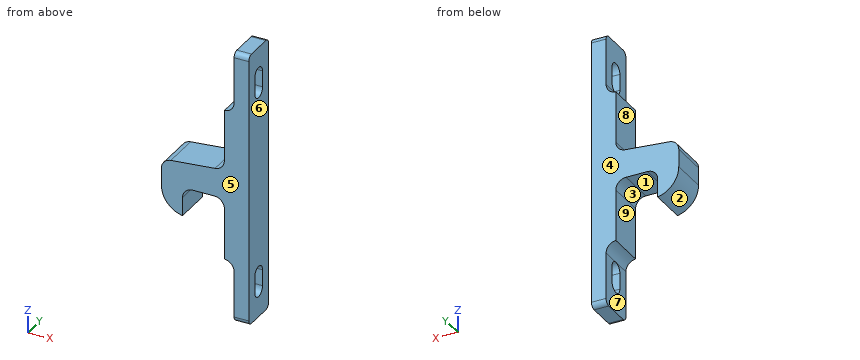
Autodesk Inventor part; units mm, degrees
ref_plane "YZ Plane" through (0, 0, 0) normal (1, 0, 0) x (0, 1, 0)
ref_plane "XZ Plane" through (0, 0, 0) normal (0, 1, 0) x (-1, 0, 0)
ref_plane "XY Plane" through (0, 0, 0) normal (0, 0, 1) x (1, 0, 0)
sketch "Boceto1" plane through (0, 0, 0) normal (0, 1, 0) x (-1, 0, 0)
  line L0 (-2.375, -26.75) -> (2.375, -26.75)
  line L1 (2.375, -26.75) -> (2.375, 26.75)
  line L2 (2.375, 26.75) -> (-2.375, 26.75)
  line L3 (-2.375, 26.75) -> (-2.375, -26.75)
  line L4 (-2.375, -26.75) -> (2.375, 26.75) construction
  line L5 (2.375, -26.75) -> (-2.375, 26.75) construction
  line L6 (2.375, 26.75) -> (0.475, 26.75)
  line L7 (0.475, 26.75) -> (0.475, 14.75)
  line L8 (0.475, 14.75) -> (2.375, 14.75)
  line L9 (2.375, 14.75) -> (2.375, 26.75)
  line L10 (2.375, -26.75) -> (0.475, -26.75)
  line L11 (0.475, -26.75) -> (0.475, -14.75)
  line L12 (0.475, -14.75) -> (2.375, -14.75)
  line L13 (2.375, -14.75) -> (2.375, -26.75)
  line L14 (2.375, -26.75) -> (2.375, -2.75)
  line L15 (2.375, -2.75) -> (10.525, -2.75)
  line L16 (10.525, -2.75) -> (10.525, -8.35)
  line L17 (10.525, -8.35) -> (14.625, -8.35)
  line L18 (14.625, -8.35) -> (14.625, 1.85)
  line L19 (14.625, 1.85) -> (2.375, 1.85)
  line L20 (14.625, 1.85) -> (2.375, 2.9217)
  point P0 (0, 0)
  point P1 (2.375, 14.75)
  point P2 (0.475, -26.75)
  point P3 (2.375, -14.75)
  dimension "d0" = 4.75
  dimension "d1" = 53.5
  dimension "d2" = 1.9
  dimension "d3" = 12
  dimension "d4" = 12
  dimension "d5" = 24
  dimension "d6" = 8.15
  dimension "d7" = 5.6
  dimension "d8" = 4.1
  dimension "d9" = 10.2
  dimension "d10" = 5
extrude "Extrusión1" add sketch "Boceto1" along normal blind 7.25 contours L3 L2 L7 L8 L1 L12 L11 L0 | L1 L19 L18 L17 L16 L15 | L1 L20 L19
fillet "Empalme1" radius 2 5 edges at (-0.475, 3.625, -14.75) (-2.375, 3.625, -2.75) (-10.525, 3.625, -2.75) (-2.375, 3.625, 2.9217) (-0.475, 3.625, 14.75)
fillet "Empalme2" radius 2 1 edges at (-14.625, 3.625, 1.85)
fillet "Empalme3" radius 5 1 edges at (-14.625, 3.625, -8.35)
fillet "Empalme4" radius 1 4 edges at (0.95, 7.25, 26.75) (0.95, 0, 26.75) (0.95, 7.25, -26.75) (0.95, 0, -26.75)
sketch "Boceto2" plane through (-0.475, 0, 16.7475) normal (-1, 0, 0) x (0, 0, 1)
  arc A0 (9.0025, 0) -> (10.0025, 1) centre (9.0025, 1) ccw
  line L0 (10.0025, 1) -> (10.0025, 6.25)
  arc A1 (10.0025, 6.25) -> (9.0025, 7.25) centre (9.0025, 6.25) ccw
  line L1 (0, 7.25) -> (9.0025, 7.25)
  line L2 (0, 0) -> (0, 7.25)
  line L3 (0, 0) -> (9.0025, 0)
  arc A2 (-43.4975, 1) -> (-42.4975, 0) centre (-42.4975, 1) ccw
  line L4 (-42.4975, 0) -> (-33.495, 0)
  line L5 (-33.495, 7.25) -> (-33.495, 0)
  line L6 (-42.4975, 7.25) -> (-33.495, 7.25)
  arc A3 (-42.4975, 7.25) -> (-43.4975, 6.25) centre (-42.4975, 6.25) ccw
  line L7 (-43.4975, 1) -> (-43.4975, 6.25)
  line L8 (4.715, 2.2) -> (2.9125, 2.2)
  line L9 (2.2, 5.05) -> (4.5775, 5.05)
  line L10 (10.0025, 3.4658) -> (6.0025, 3.4658)
  line L11 (6.0025, 3.4658) -> (6.0025, 4.2)
  line L12 (6.0025, 3.4658) -> (6.0025, 5.05)
  line L13 (4.5775, 2.2) -> (1.4275, 2.2)
  line L14 (0.0025, 3.625) -> (0.0025, 3.625)
  line L15 (1.4275, 5.05) -> (6.0025, 5.05)
  line L16 (6.0025, 3.625) -> (6.0025, 3.625)
  arc A4 (4.5775, 2.2) -> (6.0025, 3.625) centre (4.5775, 3.625) ccw
  arc A5 (6.0025, 3.625) -> (4.5775, 5.05) centre (4.5775, 3.625) ccw
  arc A6 (1.4275, 5.05) -> (0.0025, 3.625) centre (1.4275, 3.625) ccw
  arc A7 (0.0025, 3.625) -> (1.4275, 2.2) centre (1.4275, 3.625) ccw
  point P0 (-16.7475, 0)
  point P1 (6.0025, 2.2)
  point P2 (0.0025, 5.05)
  point P3 (3.715, 5.05)
  point P4 (0.0025, 3.625)
  point P5 (2.9125, 2.2)
  point P6 (4.5775, 2.2)
  point P7 (2.2, 5.05)
  dimension "d17" = 2.2
  dimension "d18" = 4
  dimension "d19" = 6
  dimension "d21" = 2.85
  dimension "d22" = 1.425
extrude "Extrusión2" cut sketch "Boceto2" against normal blind 7.25 contours L8 L13 A7 A6 L15 L9 A5 A4
ref_plane "Plano de trabajo1" through (2.375, 1, 0) normal (0, 0, -1) x (-1, 0, 0)
mirror "Simetría1" about plane through (2.375, 1, 0) normal (0, 0, -1) of "Extrusión2"
properties part number "Cierre cocina"
The model under review builds one solid part; all positions refer to its coordinate system, in mm. Face numbers are marked on the shaded views. A direction names the side the tool comes from. Give positions to 0.01 mm unless a question says otherwise; leave off trailing zeros. Loops run counter-clockwise (first coordinate to the right, second up) from the corner with the lowest first, then second, coordinate; pieces in that order, holes last. Notation, with made-up numbers: (22, -20.75) -> (74, -20.75) arc R23 cw to (74, -8.75) -> close; hole circle Ø9 at (11.5, 13.25). An arc over 180 degrees is marked (long way). Write each question's results on one line, items separated by ' | '.
1) Take a section at C-C, the plane z = 22. Give the boundary of the cut face in (x, y) (3 decimals).
Conclusion:
outline: (-0.475, 0) -> (2.375, 0) -> (2.375, 2.37) -> (-0.475, 2.37) -> close; (-0.475, 4.88) -> (2.375, 4.88) -> (2.375, 7.25) -> (-0.475, 7.25) -> close
2) Take a section at D-D, the plane x = -11. Give the boundary of the cut face in (y, z).
Conclusion:
outline: (0, -8.24) -> (7.25, -8.24) -> (7.25, 2.17) -> (0, 2.17) -> close
3) Draft analysis for pull direction X (two halves, no side actions). For the marked faces 1, 2, 3 and 4, state which applies: pulls with the +X half, pulls with the -X half, needs draft (parallel to the pull), parting line crosses it, or undercut.
Conclusion:
face 1: undercut | face 2: pulls with the -X half | face 3: undercut | face 4: needs draft
4) Insertion check: pin 1 Ø2 at (x, y) = (-4.5, 4) entering from +Z; pin 2 Ø1.2 at (x, y) = (-5.5, 5) entering from -Z; pin 3 Ø3.5 at (y, z) = (5, 20) entering from -X (3 decimals). Each pin has a flat end and moves straight along its axis. Give the tip position at first contact, or say it passes through.
Conclusion:
pin 1: stops at z = 2.96 | pin 2: stops at z = -2.75 | pin 3: stops at x = -0.475
5) Tool access review of the marked faces 5, 6, 7, 8 and 9: name each direction out of +Z, -Z, +X, -X, +Y, -Y from which nothing blocks a thin tool from reaching the whole face with its end or side.
Conclusion:
face 5: +Z, -Z, +X, -X, -Y | face 6: +Z, -Z, +X, +Y, -Y | face 7: -Z, -X, +Y, -Y | face 8: +Z, -X, +Y, -Y | face 9: -Z, +Y, -Y
6) Take a section at A-A, the plane z = -19.5. Give the boundary of the cut face in (x, y) (3 decimals), plus the area to 3 significant figures.
Conclusion:
outline: (-0.475, 0) -> (2.375, 0) -> (2.375, 2.2) -> (-0.475, 2.2) -> close; (-0.475, 5.05) -> (2.375, 5.05) -> (2.375, 7.25) -> (-0.475, 7.25) -> close | area: 12.5 mm^2
7) For line 1 along Y through (x, z) = (1.25, 18.5); line 2 along X through (y, z) = (3.5, -13) (3 decimals); line 3 along X through (y, z) = (5.25, 17.5) (3 decimals), list the stretches that pass through material, from the lowest coordinate up. Write a range as from..to.
Conclusion:
line 1: y = 0..2.2, 5.05..7.25 | line 2: x = -2.375..2.375 | line 3: x = -0.475..2.375
